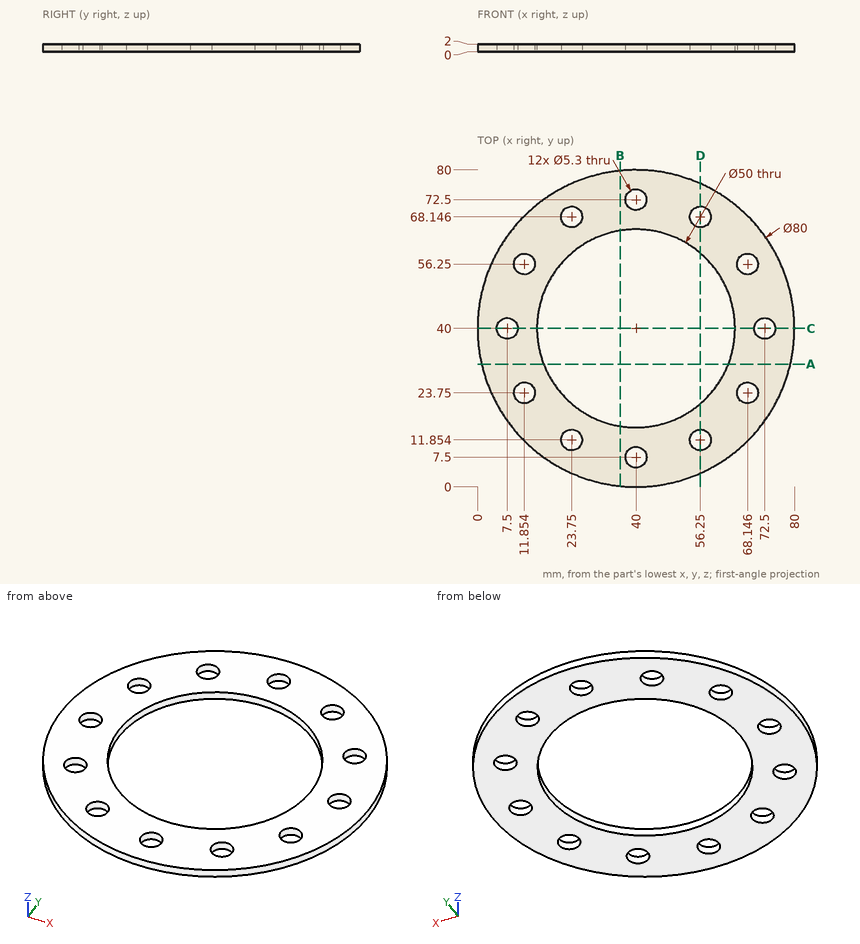
Source: three-view drawing plus pictorial views. Frame: mm from the lowest corner of the part. Coordinates: 2 decimals unless noted, no trailing zeros. Loops run counter-clockwise (first coordinate to the right, second up) from the corner with the lowest first, then second, coordinate; pieces in that order, holes last. Notation, with made-up numbers: (7, 45.5) -> (54, 45.5) arc R21 ccw to (54, 54.5) -> close; hole circle Ø3 at (47, -35). An arc over 180 degrees is marked (long way). One line per item, written item: value.
(1) Cut plane A-A (y = 31). Output: boundary loops of the cut face in (x, z), then the cut area to 3 significant figures.
Answer below:
outline: (1.03, 0) -> (16.68, 0) -> (16.68, 2) -> (1.03, 2) -> close; (63.32, 0) -> (78.97, 0) -> (78.97, 2) -> (63.32, 2) -> close
area: 62.6 mm2
(2) Cut plane D-D (x = 56.25). Output: boundary loops of the cut face in (y, z).
Answer below:
outline: (3.45, 0) -> (9.2, 0) -> (9.2, 2) -> (3.45, 2) -> close; (14.5, 0) -> (21, 0) -> (21, 2) -> (14.5, 2) -> close; (59, 0) -> (65.5, 0) -> (65.5, 2) -> (59, 2) -> close; (70.8, 0) -> (76.55, 0) -> (76.55, 2) -> (70.8, 2) -> close
(3) Ray query, line 1 along Y through (x, z) = (13, 1.3); line 2 along X through (y, z) = (39, 0.55); line 3 along Y through (x, z) = (23.5, 1). Return the intervals inside material, ascending.
Answer below:
line 1: y = 10.49 to 21.36, 26.14 to 53.86, 58.64 to 69.51
line 2: x = 0.01 to 5.05, 9.95 to 15.02, 64.98 to 70.05, 74.95 to 79.99
line 3: y = 3.56 to 9.22, 14.49 to 21.22, 58.78 to 65.51, 70.78 to 76.44
(4) Cut plane C-C (y = 40). Output: boundary loops of the cut face in (x, z).
Answer below:
outline: (0, 0) -> (4.85, 0) -> (4.85, 2) -> (0, 2) -> close; (10.15, 0) -> (15, 0) -> (15, 2) -> (10.15, 2) -> close; (65, 0) -> (69.85, 0) -> (69.85, 2) -> (65, 2) -> close; (75.15, 0) -> (80, 0) -> (80, 2) -> (75.15, 2) -> close
(5) Cut plane B-B (x = 36). Output: boundary loops of the cut face in (y, z), then the cut area to 3 significant figures.
Answer below:
outline: (0.2, 0) -> (15.32, 0) -> (15.32, 2) -> (0.2, 2) -> close; (64.68, 0) -> (79.8, 0) -> (79.8, 2) -> (64.68, 2) -> close
area: 60.5 mm2
(6) Pin query (flat end, axial travel): pin 1 Ø4 at (x, y) = (23.75, 68.15) entering from -Z; pin 2 Ø1 at (x, z) = (12.5, 0.5) entering from +Y. Return the tip coordinate at first contact, or that it passes through.
Answer below:
pin 1: passes through
pin 2: stops at y = 69.51
